from build123d import *

# Parameters (mm, degrees)
F1_DEPTH      = 19.05
F3_DEPTH      = 5.5993816375
F3_DEPTH_BACK = 40.1226183625
F5_DEPTH      = 14.0315074599
F6_R          = 2.54


with BuildPart() as f1:
    # F0 (on Right) → F1 (new body, symmetric)
    with BuildSketch(Plane.YZ):
        with BuildLine():
            ThreePointArc((0.4305788672, -2.4419341014), (0.2003852832, 0.0026537646), (0.365760616, 2.4524802728))
            Line((0.365760616, 2.4524802728), (5.5983816375, 37.5379959634))
            Line((5.5983816375, 37.5379959634), (1.8300595357, 38.1))
            Line((1.8300595357, 38.1), (-3.5937905479, 1.7322645138))
            ThreePointArc((-3.5937905479, 1.7322645138), (-4.276919676, 0.4928303362), (-5.6035623355, 0))
            Line((-5.6035623355, 0), (-40.1216183625, 0))
            Line((-40.1216183625, 0), (-40.1216183625, -3.175))
            Line((-40.1216183625, -3.175), (-35.0830748888, -3.175))
            Line((-35.0830748888, -3.175), (-40.1216183625, -31.75))
            Line((-40.1216183625, -31.75), (-33.7716183625, -31.75))
            Line((-33.7716183625, -31.75), (-30.6699266617, -23.2281720899))
            ThreePointArc((-30.6699266617, -23.2281720899), (-28.3450888905, -20.1983845188), (-24.7028785197, -19.05))
            Line((-24.7028785197, -19.05), (-9.8203582053, -19.05))
            ThreePointArc((-9.8203582053, -19.05), (-6.1781478345, -20.1983845188), (-3.8533100633, -23.2281720899))
            Line((-3.8533100633, -23.2281720899), (-0.7516183625, -31.75))
            Line((-0.7516183625, -31.75), (5.5983816375, -31.75))
            Line((5.5983816375, -31.75), (0.4305788672, -2.4419341014))
        make_face()
    extrude(amount=F1_DEPTH, both=True)

    # F2 (on Front) → F3 (cut, two sides)
    with BuildSketch(Plane.XZ) as f3_sk:
        with BuildLine():
            Line((-9.5983082992, -23.2281720899), (-12.7, -31.75))
            Line((-12.7, -31.75), (0, -31.75))
            Line((0, -31.75), (12.7, -31.75))
            Line((12.7, -31.75), (9.5983082992, -23.2281720899))
            ThreePointArc((9.5983082992, -23.2281720899), (7.273470528, -20.1983845188), (3.6312601572, -19.05))
            Line((3.6312601572, -19.05), (0, -19.05))
            Line((0, -19.05), (-3.6312601572, -19.05))
            ThreePointArc((-3.6312601572, -19.05), (-7.273470528, -20.1983845188), (-9.5983082992, -23.2281720899))
        make_face()
    extrude(amount=-F3_DEPTH, mode=Mode.SUBTRACT)
    extrude(f3_sk.sketch, amount=F3_DEPTH_BACK, mode=Mode.SUBTRACT)

    # F4 (on face) → F5 (cut, through all)
    with BuildSketch(Plane(origin=(0, -3.7683221018, 0.5620040366), x_dir=(1, 0, 0), z_dir=(0, -0.9890609191, 0.1475076212))):
        with BuildLine():
            ThreePointArc((0, 27.3717801606), (-4.4901280605, 25.5119082211), (-6.35, 21.0217801606))
            Line((-6.35, 21.0217801606), (-6.35, 15.9417801606))
            ThreePointArc((-6.35, 15.9417801606), (-4.4901280605, 11.4516521), (0, 9.5917801606))
            ThreePointArc((0, 9.5917801606), (4.4901280605, 11.4516521), (6.35, 15.9417801606))
            Line((6.35, 15.9417801606), (6.35, 21.0217801606))
            ThreePointArc((6.35, 21.0217801606), (4.4901280605, 25.5119082211), (0, 27.3717801606))
        make_face()
    extrude(amount=-F5_DEPTH, mode=Mode.SUBTRACT)

    # F6
    f6_edges = [f1.edges().sort_by_distance(p)[0] for p in [
        (19.05, 3.714221, 37.818998),
        (-19.05, 3.714221, 37.818998),
        (-19.05, -40.121618, -1.5875),
        (19.05, -40.121618, -1.5875),
    ]]
    fillet(f6_edges, radius=F6_R)


solid = f1.part
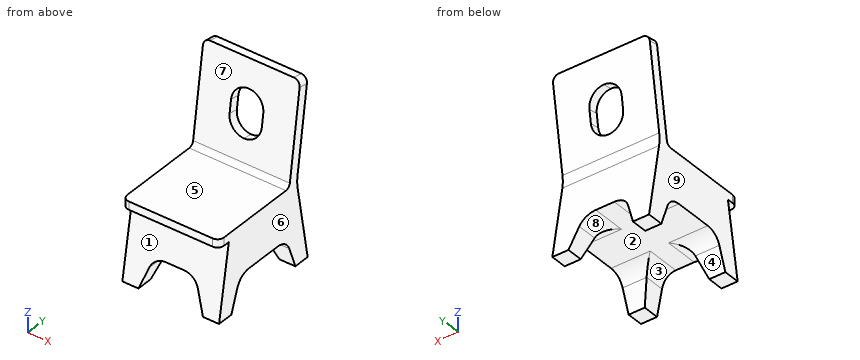
Input: part model. Units: mm. Frame: model coordinates. Face numbers are marked on the shaded views. A direction names the side the tool comes from. Coordinates: 2 decimals unless noted, no trailing zeros. Loops run counter-clockwise (first coordinate to the right, second up) from the corner with the lowest first, then second, coordinate; pieces in that order, holes last. Notation, with made-up numbers: (54.5, 83.5) - (81.5, 83.5) arc R26 ccw to (81.5, 118.5) - close; hole circle Ø8 at (3.5, 19). An arc over 180 degrees is marked (long way). Answer in a Markdown table with one row per item. Add a question column.
Item 1: Section query C-C on y = -29.5. Return the cut outline in (x, z), then the cut area to 3 significant figures.
Item 2: Section query A-A on x = -13.5. Return the cut outline in (y, z) (3 decimals), then the cut area to 3 significant figures.
Item 3: Section query B-B on x = -5.5. Return the cut outline in (y, z) (3 decimals).
Item 4: Mould query, pull axis X, two halves, no side actions, for the marked faces 6, 7, 8 and 9. Classes: released by +X, released by -X, zero draft, split by the parting line, or undercut.
Item 5: Access query for the marked faces 1, 2, 3, 4 and 5. Directions: +Z, -Z, +X, -X, +Y, -Y. A direction counts if a zero-diameter tool reaches every point of the face in a straight line with its end or side. Return the directions, or none.
Item 6: Line query: line 1 along Z through (x, y) = (-1, -28); line 2 along X through (y, z) = (3.5, -27.5); line 3 along Y through (x, z) = (-14.5, -4). Output: solid intervals per line, ascending. Write a range as [from, to].
Item 7: Section query D-D on z = 7.5. Return the cut outline in (x, y).
Item 8: Contact query for flat-ended pins moving along their axis: P1, Ø12, axis at x = -1.5, y = -31.5, coming from the -Z side; P2, Ø19, axis at x = 8.5, y = -14.5, coming from the -Z side; P3, Ø8, axis at x = 5.5, z = 28, coming from the +Y side. Output: stop coordinate, or through.
Recorded:
| question | item | result |
|---|---|---|
| 1 | outline | (-19.05, -21.24) - (-8.43, -21.24) arc R6.35 cw to (-3.63, -19.05) - (3.63, -19.05) arc R6.35 cw to (8.43, -21.24) - (19.05, -21.24) - (19.05, 0) - (-19.05, 0) - close |
| 1 | area | 779 mm^2 |
| 2 | outline | (-40.122, -31.75) - (-33.772, -31.75) - (-30.67, -23.228) arc R6.35 cw to (-24.703, -19.05) - (-9.82, -19.05) arc R6.35 cw to (-3.853, -23.228) - (-0.752, -31.75) - (5.598, -31.75) - (0.431, -2.442) arc R15.24 cw to (0.366, 2.452) - (5.598, 37.538) - (1.83, 38.1) - (-3.594, 1.732) arc R2.032 cw to (-5.604, 0) - (-40.122, 0) - (-40.122, -3.175) - (-35.083, -3.175) - close |
| 2 | area | 1,080 mm^2 |
| 3 | outline | (-40.122, -3.175) - (-35.083, -3.175) - (-37.932, -19.331) - (-26.572, -19.331) arc R6.35 cw to (-24.703, -19.05) - (-9.82, -19.05) arc R6.35 cw to (-7.952, -19.331) - (3.409, -19.331) - (0.431, -2.442) arc R15.24 cw to (0.366, 2.452) - (1.883, 12.628) - (-1.885, 13.19) - (-3.594, 1.732) arc R2.032 cw to (-5.604, 0) - (-40.122, 0) - close; (-0.199, 24.493) - (3.569, 23.931) - (5.598, 37.538) - (1.83, 38.1) - close |
| 4 | face 6 | released by +X |
| 4 | face 7 | zero draft |
| 4 | face 8 | undercut |
| 4 | face 9 | released by -X |
| 5 | face 1 | +X, -X, -Y |
| 5 | face 2 | -Z |
| 5 | face 3 | -Z, +Y, -Y |
| 5 | face 4 | -Z, +X, -X |
| 5 | face 5 | +Z, +X, -X, -Y |
| 6 | line 1 | [-19.05, 0] |
| 6 | line 2 | [-19.05, -11.15], [11.15, 19.05] |
| 6 | line 3 | [-35.23, 0.71] |
| 7 | outline | (-19.05, -2.73) - (19.05, -2.73) - (19.05, 1.12) - (-19.05, 1.12) - close |
| 8 | P1 | z = -20.36 |
| 8 | P2 | z = -21.27 |
| 8 | P3 | y = 4.77 |
